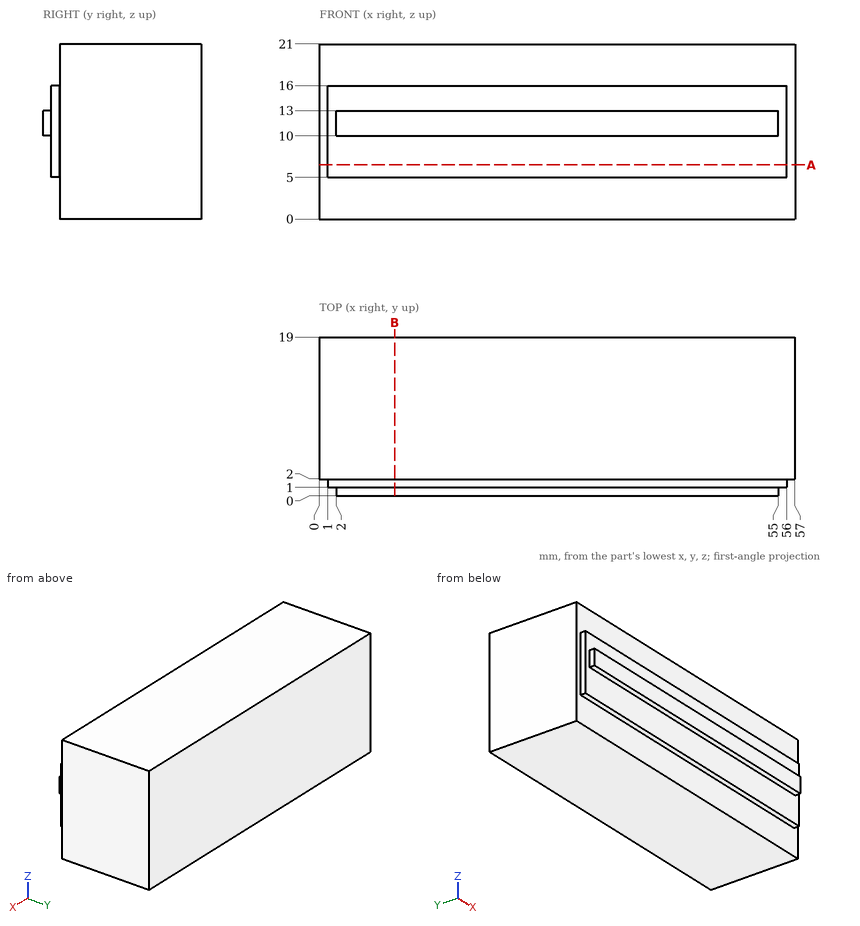
Here's the drawing with two shaded views (mm, measured from the low corner). I have some questions. Coordinates: 2 decimals unless noted, no trailing zeros. Loops run counter-clockwise (first coordinate to the right, second up) from the corner with the lowest first, then second, coordinate; pieces in that order, holes last.
Item 1: Suppose I cut it at A-A (z = 6.5). Please give me the cut outline in (x, y).
Answers below:
outline: (0, 2) - (1, 2) - (1, 1) - (56, 1) - (56, 2) - (57, 2) - (57, 19) - (0, 19) - close
Item 2: I'm going to push flat-ended pins straight in: pin 1 (1.1 mm diameter, centred on x = 22, y = 0.5, fed in from -Z); pin 2 (0.8 mm diameter, centred on x = 27.5, y = 1.5, fed in from +Z); pin 3 (0.8 mm diameter, centred on x = 34, y = 0.5, fed in from +Z). Where does each tip first touch, or does it pass through?
Answers below:
pin 1: stops at z = 5
pin 2: stops at z = 16
pin 3: stops at z = 13
Item 3: Suppose I cut it at B-B (x = 9). Please give me the cut outline in (y, z), then the cut area to 3 significant figures.
Answers below:
outline: (0, 10) - (1, 10) - (1, 5) - (2, 5) - (2, 0) - (19, 0) - (19, 21) - (2, 21) - (2, 16) - (1, 16) - (1, 13) - (0, 13) - close
area: 371 mm2
Item 4: Please list where these lines run through material, in increasing order: L1, parallel to Y at x = 52.5, z = 15.5; L2, parallel to Y at x = 23.5, z = 18.75; L3, parallel to X at y = 1.25, z = 7.75.
Answers below:
L1: y = 1 to 19
L2: y = 2 to 19
L3: x = 1 to 56
